```python
from build123d import *

# Parameters (mm, degrees)
SKETCH1_W           = 40
SKETCH1_H           = 45
BOSS_EXTRUDE1_DEPTH = 30
SKETCH2_R           = 8
CUT_EXTRUDE1_DEPTH  = 55.829280499
SKETCH3_R           = 3
CUT_EXTRUDE2_DEPTH  = 43.5


with BuildPart() as part:
    # Sketch1 → Boss-Extrude1 (new body)
    with BuildSketch(Plane.XY):
        Rectangle(SKETCH1_W, SKETCH1_H)
    extrude(amount=BOSS_EXTRUDE1_DEPTH)

    # Sketch2 → Cut-Extrude1 (cut, through all)
    with BuildSketch(Plane(origin=(20, 0, 0), x_dir=(0, 0, -1), z_dir=(1, 0, 0))):
        with Locations(Location((-16, 0, 0), (0, 0, 90))):
            Circle(SKETCH2_R)
    extrude(amount=-CUT_EXTRUDE1_DEPTH, mode=Mode.SUBTRACT)

    # Sketch3 → Cut-Extrude2 (cut, through all)
    with BuildSketch(Plane.XY.offset(30)):
        with Locations((-12.5, 16)):
            Circle(SKETCH3_R)
        with Locations((12.5, 16)):
            Circle(SKETCH3_R)
        with Locations((12.5, -16)):
            Circle(SKETCH3_R)
        with Locations((-12.5, -16)):
            Circle(SKETCH3_R)
    extrude(amount=-CUT_EXTRUDE2_DEPTH, mode=Mode.SUBTRACT)


solid = part.part
```
Read the model definition and answer for the solid it produces. Units are mm, in the model's axes. Coordinates: 2 decimals unless noted, no trailing zeros. Write each loop counter-clockwise with the first axis right and the second up, starting at its lowest first coordinate (ties: lowest second). Pieces come first, ordered by that corner, then holes. Notation, with made-up numbers: (-8, 34) -> (41, 34) arc R21 ccw to (41, 38) -> close; hole circle Ø1 at (69, 32.5). An arc over 180 degrees is marked (long way). Write item = value, one per line.
(1) Straight lines are drawn through the part: L1, parallel to Y at x = -12.5, z = 6.5; L2, parallel to Y at x = 12.5, z = 9.5; L3, parallel to Y at x = 14.5, z = 9. For each, find the intervals that lie inside material, in ascending order. Write a range as from..to.
From the geometry:
L1 = -22.5..-19, -13..13, 19..22.5
L2 = -22.5..-19, -13..-4.66, 4.66..13, 19..22.5
L3 = -22.5..-18.24, -13.76..-3.87, 3.87..13.76, 18.24..22.5
(2) For a pull along Y with two mould halves and no side action, classify faces 1 (the face through (20, -5, 8)), 2 (the face through (-14.9, 14.2, 15.2)), 3 (the face through (0, -22.5, 15)) as +Y half, -Y half, draft (parallel to the pull), parting line (faces both ways), or undercut.
From the geometry:
face_1 = draft
face_2 = undercut
face_3 = -Y half
(3) Section B-B on x = 12.5 is taken. Write down the section's boundary in (y, z), plus the area to 3 significant figures.
From the geometry:
outline = (-22.5, 0) -> (-19, 0) -> (-19, 30) -> (-22.5, 30) -> close; (-13, 0) -> (13, 0) -> (13, 30) -> (-13, 30) -> close; (19, 0) -> (22.5, 0) -> (22.5, 30) -> (19, 30) -> close; hole circle Ø16 at (0, 16)
area = 789 mm2
(4) Section D-D on y = -16 is taken. Write down the section's boundary in (x, z), plus the area to 3 significant figures.
From the geometry:
outline = (-20, 0) -> (-15.5, 0) -> (-15.5, 30) -> (-20, 30) -> close; (-9.5, 0) -> (9.5, 0) -> (9.5, 30) -> (-9.5, 30) -> close; (15.5, 0) -> (20, 0) -> (20, 30) -> (15.5, 30) -> close
area = 840 mm2
(5) Section A-A on z = 16 is taken. Write down the section's boundary in (x, y), plus the area to 3 significant figures.
From the geometry:
outline = (-20, -22.5) -> (20, -22.5) -> (20, -8) -> (-20, -8) -> close; (-20, 8) -> (20, 8) -> (20, 22.5) -> (-20, 22.5) -> close; hole circle Ø6 at (-12.5, -16); hole circle Ø6 at (-12.5, 16); hole circle Ø6 at (12.5, -16); hole circle Ø6 at (12.5, 16)
area = 1,050 mm2
(6) Section C-C on y = 0 is taken. Write down the section's boundary in (x, z).
From the geometry:
outline = (-20, 0) -> (20, 0) -> (20, 8) -> (-20, 8) -> close; (-20, 24) -> (20, 24) -> (20, 30) -> (-20, 30) -> close
